Input: dimensioned drawing with shaded views. Units: mm. Origin: part minimum x, y, z. Give positions to 0.01 mm unless a question says otherwise; leave off trailing zeros. Loops run counter-clockwise (first coordinate to the right, second up) from the corner with the lowest first, then second, coordinate; pieces in that order, holes last.
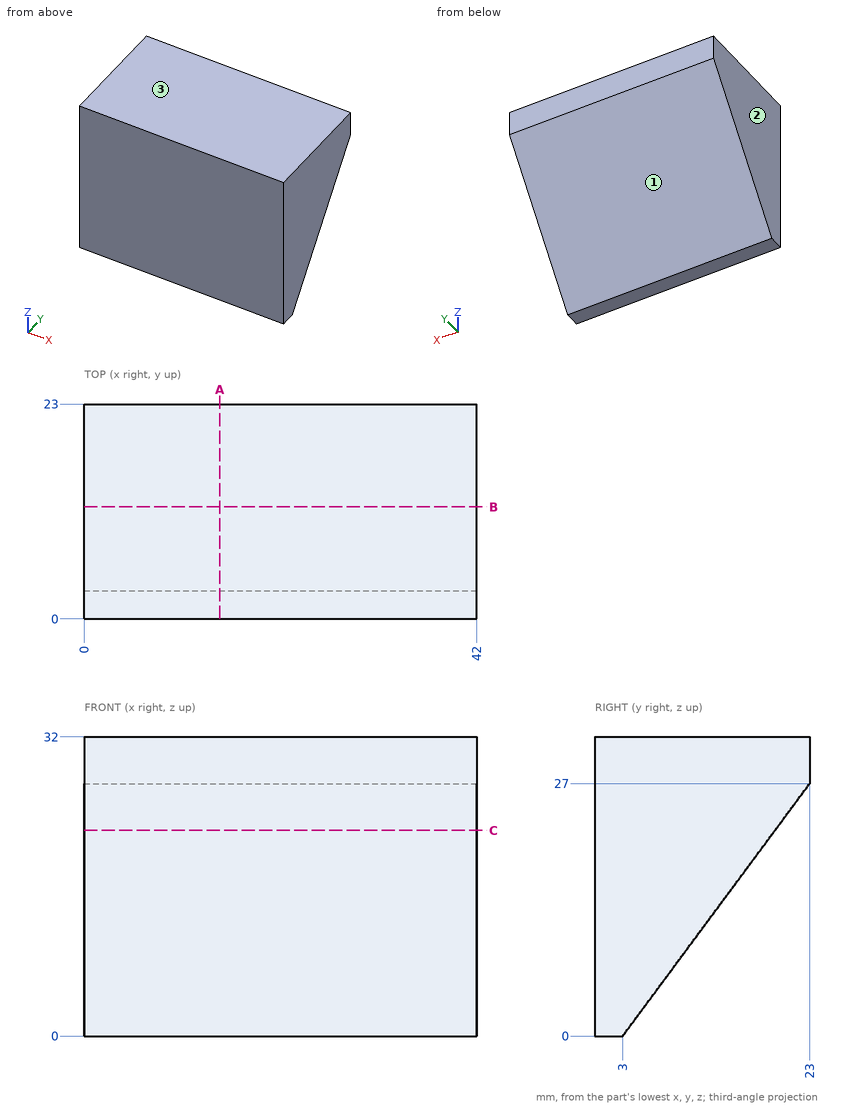
(1) Section B-B, the plane y = 12. Return the cut outline in (x, z).
A:
outline: (0, 12.15) - (42, 12.15) - (42, 32) - (0, 32) - close
(2) Section A-A, the plane x = 14.5. Return the cut outline in (y, z).
A:
outline: (0, 0) - (3, 0) - (23, 27) - (23, 32) - (0, 32) - close
(3) Ray query, line 1 along Z through (x, y) = (26.5, 10.75); line 2 along Y through (x, z) = (40, 24); line 3 along Z through (x, y) = (8.5, 4.75). Return the intervals inside material, ascending.
A:
line 1: z = 10.46 to 32
line 2: y = 0 to 20.78
line 3: z = 2.36 to 32
(4) Section C-C, the plane z = 22. Return the cut outline in (x, y), then the cut area to 3 significant figures.
A:
outline: (0, 0) - (42, 0) - (42, 19.3) - (0, 19.3) - close
area: 810 mm2
(5) First-contact query: pin 1 (5 mm diameter, centred on x = 5, z = 5.5, fed in from +Y); pin 2 (6 mm diameter, centred on x = 28.5, y = 13, fed in from -Z); pin 3 (5 mm diameter, centred on x = 12, y = 18, fed in from -Z) (3 decimals). Flat tips, straight axial feed; report the tip coordinate or a pass-through.
A:
pin 1: stops at y = 8.93
pin 2: stops at z = 9.45
pin 3: stops at z = 16.875
(6) Mould query, pull axis Z, two halves, no side actions, for the marked faces 1, 2 and 3. Classes: pulls with the +Z half, pulls with the -Z half, needs draft (parallel to the pull), parting line crosses it, or undercut.
A:
face 1: pulls with the -Z half
face 2: needs draft
face 3: pulls with the +Z half
